Model file for the job. Use its own axes, mm. Give positions to 0.01 mm unless a question says otherwise; leave off trailing zeros. Loops run counter-clockwise (first coordinate to the right, second up) from the corner with the lowest first, then second, coordinate; pieces in that order, holes last. Notation, with made-up numbers: (25, 23.25) -> (48, 23.25) arc R22 cw to (48, 32.25) -> close; hole circle Ø11 at (34, 18.25). An arc over 180 degrees is marked (long way). Use CSV: the item, a comma, the result in double quotes. Start each with the question number.
(1) Flat gauge pins, fed straight in: pin 1 (1 mm diameter, centred on y = 7, z = 7, fed in from +X); pin 2 (3 mm diameter, centred on y = 2.5, z = -8.5, fed in from +X); pin 3 (11 mm diameter, centred on x = -134.5, z = 2, fed in from +Y); pin 4 (3 mm diameter, centred on x = 8, z = 0, fed in from -Y). Where does each tip first touch, or does it go through?
(2) Cut at A-A on x = -49. Write the cut outline in (y, z).
(3) Drill centre lines: probe 1 along Z at (x, y) = (0, 7.25); probe 2 along X at (y, z) = (7.25, 0); probe 3 along Z at (x, y) = (0, 5.5). Where is each one in solid material? Low to high.
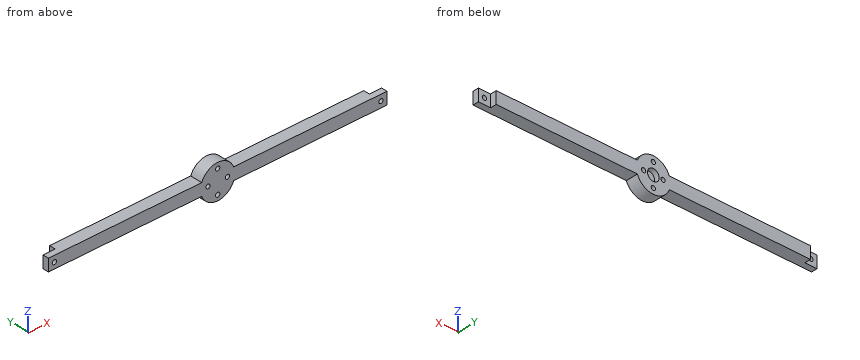
from build123d import *

# Parameters (mm, degrees)
SKETCH1_R           = 14
BOSS_EXTRUDE1_DEPTH = 10
BOSS_EXTRUDE2_DEPTH = 10
CUT_EXTRUDE2_DEPTH  = 20
SKETCH6_R           = 1.75
CUT_EXTRUDE4_DEPTH  = 10
CIRPATTERN2_COUNT   = 2
CIRPATTERN2_ANGLE   = 180
SKETCH5_R           = 1.75
CUT_EXTRUDE3_DEPTH  = 11
SKETCH7_R           = 4.75
CUT_EXTRUDE5_DEPTH  = 4


with BuildPart() as part:
    # Sketch1 → Boss-Extrude1 (new body)
    with BuildSketch(Plane(origin=(0, 0, 0), x_dir=(1, 0, 0), z_dir=(0, 1, 0))):
        Circle(SKETCH1_R)
    extrude(amount=BOSS_EXTRUDE1_DEPTH)

    # Sketch2 → Boss-Extrude2 (add)
    with BuildSketch(Plane(origin=(0, 10, 0), x_dir=(1, 0, 0), z_dir=(0, 1, 0))):
        with BuildLine():
            Line((13.076696831, -5), (149, -5))
            Line((149, -5), (149, 5))
            Line((149, 5), (13.076696831, 5))
            ThreePointArc((13.076696831, 5), (14, 0), (13.076696831, -5))
        make_face()
    boss_extrude2 = extrude(amount=-BOSS_EXTRUDE2_DEPTH)

    # Sketch4 → Cut-Extrude2 (cut, through all)
    with BuildSketch(Plane.XY.offset(5)):
        Polygon((138.9, 0), (138.9, 4.9), (128.9, 4.9), (128.9, 10), (149, 10), (149, 0), align=None)
    cut_extrude2 = extrude(amount=-CUT_EXTRUDE2_DEPTH, mode=Mode.SUBTRACT)

    # Sketch6 → Cut-Extrude4 (cut)
    with BuildSketch(Plane(origin=(0, 4.9, 0), x_dir=(1, 0, 0), z_dir=(0, 1, 0))):
        with Locations((134, 0)):
            Circle(SKETCH6_R)
    cut_extrude4 = extrude(amount=-CUT_EXTRUDE4_DEPTH, mode=Mode.SUBTRACT)

    # CirPattern2: Boss-Extrude2, Cut-Extrude2, Cut-Extrude4 ×2 about axis
    cirpattern2_axis = Axis((0, 0, 0), (0, 1, 0))
    for i in range(1, CIRPATTERN2_COUNT):
        add(boss_extrude2.rotate(cirpattern2_axis, i * CIRPATTERN2_ANGLE / (CIRPATTERN2_COUNT - 1)))
        add(cut_extrude2.rotate(cirpattern2_axis, i * CIRPATTERN2_ANGLE / (CIRPATTERN2_COUNT - 1)), mode=Mode.SUBTRACT)
        add(cut_extrude4.rotate(cirpattern2_axis, i * CIRPATTERN2_ANGLE / (CIRPATTERN2_COUNT - 1)), mode=Mode.SUBTRACT)

    # Sketch5 → Cut-Extrude3 (cut, through all)
    with BuildSketch(Plane(origin=(0, 10, 0), x_dir=(1, 0, 0), z_dir=(0, 1, 0))):
        with Locations((0, 9.5)):
            Circle(SKETCH5_R)
        with Locations((8, 0)):
            Circle(SKETCH5_R)
        with Locations((-8, 0)):
            Circle(SKETCH5_R)
        with Locations((0, -9.5)):
            Circle(SKETCH5_R)
    extrude(amount=-CUT_EXTRUDE3_DEPTH, mode=Mode.SUBTRACT)

    # Sketch7 → Cut-Extrude5 (cut)
    with BuildSketch(Plane(origin=(0, 10, 0), x_dir=(1, 0, 0), z_dir=(0, 1, 0))):
        Circle(SKETCH7_R)
    extrude(amount=-CUT_EXTRUDE5_DEPTH, mode=Mode.SUBTRACT)


solid = part.part
Check result:
1,pin 1,"x = 12.4"
1,pin 2,"x = 12.12"
1,pin 3,"y = 4.9"
1,pin 4,"through"
2,outline,"(0, -5) -> (10, -5) -> (10, 5) -> (0, 5) -> close"
3,probe 1,"-14 to -11.25, -7.75 to -4.75, 4.75 to 7.75, 11.25 to 14"
3,probe 2,"-128.9 to -9.75, -6.25 to -4.75, 4.75 to 6.25, 9.75 to 128.9"
3,probe 3,"-14 to -11.25, -7.75 to 7.75, 11.25 to 14"
